from build123d import *

# Parameters (mm, degrees)
BOSS_EXTRUDE1_DEPTH = 5
SKETCH1_3_W         = 10
SKETCH1_3_H         = 5
BOSS_EXTRUDE2_DEPTH = 9
SKETCH2_W           = 40
SKETCH2_H           = 3.955098896
BOSS_EXTRUDE4_DEPTH = 12.5
FILLET1_R           = 2
SKETCH6_R           = 1.6
CUT_EXTRUDE1_DEPTH  = 3.955098897
FILLET2_R           = 1
FILLET3_R           = 2


with BuildPart() as part:
    # Sketch1 → Boss-Extrude1 (new body)
    with BuildSketch(Plane(origin=(0, 0, 0), x_dir=(1, 0, 0), z_dir=(0, 1, 0))):
        Polygon((-4.61462686, -18.720861087), (-14.61462686, -18.720861087), (-14.61462686, -25.920861087), (-34.61462686, -25.920861087), (-34.61462686, -18.720861087), (-44.61462686, -18.720861087), (-44.61462686, -35.875959983), (-4.61462686, -35.875959983), align=None)
    extrude(amount=BOSS_EXTRUDE1_DEPTH)

    # Sketch1<3> → Boss-Extrude2 (add)
    with BuildSketch(Plane(origin=(0, 0, 0), x_dir=(1, 0, 0), z_dir=(0, 1, 0))):
        with Locations((-39.61462686, -21.220861087)):
            Rectangle(SKETCH1_3_W, SKETCH1_3_H)
        with Locations((-9.61462686, -21.220861087)):
            Rectangle(SKETCH1_3_W, SKETCH1_3_H)
    extrude(amount=BOSS_EXTRUDE2_DEPTH)

    # Sketch2 → Boss-Extrude4 (add)
    with BuildSketch(Plane(origin=(0, 5, 0), x_dir=(1, 0, 0), z_dir=(0, 1, 0))):
        with Locations((-24.61462686, -33.898410535)):
            Rectangle(SKETCH2_W, SKETCH2_H)
    extrude(amount=BOSS_EXTRUDE4_DEPTH)

    # Fillet1
    fillet1_edges = [part.edges().sort_by_distance(p)[0] for p in [
        (-34.61462686, 0, 22.320861087),
        (-24.61462686, 0, 25.920861087),
        (-14.61462686, 0, 22.320861087),
        (-9.61462686, 0, 18.720861087),
        (-4.61462686, 0, 27.298410535),
        (-24.61462686, 0, 35.875959983),
        (-44.61462686, 0, 27.298410535),
        (-44.61462686, 4.5, 18.720861087),
        (-34.61462686, 4.5, 18.720861087),
        (-14.61462686, 4.5, 18.720861087),
        (-4.61462686, 4.5, 18.720861087),
        (-4.61462686, 8.75, 35.875959983),
        (-44.61462686, 8.75, 35.875959983),
        (-24.61462686, 5, 25.920861087),
        (-39.61462686, 9, 18.720861087),
        (-44.61462686, 9, 21.220861087),
        (-34.61462686, 9, 21.220861087),
        (-14.61462686, 9, 21.220861087),
        (-4.61462686, 9, 21.220861087),
        (-9.61462686, 9, 18.720861087),
        (-39.61462686, 0, 18.720861087),
    ]]
    fillet(fillet1_edges, radius=FILLET1_R)

    # Sketch6 → Cut-Extrude1 (cut)
    with BuildSketch(Plane(origin=(0, 0, 31.920861087), x_dir=(-1, 0, 0), z_dir=(0, 0, -1))):
        with Locations((24.61462686, 12)):
            Circle(SKETCH6_R)
    extrude(amount=-CUT_EXTRUDE1_DEPTH, mode=Mode.SUBTRACT)

    # Fillet2
    fillet2_edges = [part.edges().sort_by_distance(p)[0] for p in [
        (-23.01462686, 12, 31.920861087),
        (-23.01462686, 12, 35.875959984),
    ]]
    fillet(fillet2_edges, radius=FILLET2_R)

    # Fillet3
    fillet3_edges = [part.edges().sort_by_distance(p)[0] for p in [
        (-24.61462686, 17.5, 31.920861087),
    ]]
    fillet(fillet3_edges, radius=FILLET3_R)


solid = part.part
Design review of the part built by this model. Coordinates are the model's own, in mm. A direction names the side the tool comes from. Round coordinates to 2 decimals unless told otherwise and drop trailing zeros. Write each loop counter-clockwise with the first axis right and the second up, starting at its lowest first coordinate (ties: lowest second). Pieces come first, ordered by that corner, then holes.
Item 1: Consider section B-B on y = 6. Give the boundary of the cut face in (x, z), and give its area (3 significant figures).
Item 2: For pin 1 Ø10 at (x, z) = (-10, 28.5) entering from +Y; pin 2 Ø0.5 at (x, y) = (-23, 2.5) entering from -Z; pin 3 Ø8 at (x, y) = (-18, 13.5) entering from -Z, all flat-tipped, find the tip position at first contact; note any pin that passes through.
Item 3: Consider section D-D on y = 15. Give the boundary of the cut face in (x, z).
Item 4: Consider section C-C on x = -29.5. Give the boundary of the cut face in (y, z), and give its area (3 significant figures).
Item 5: Consider section A-A on y = 12. Give the boundary of the cut face in (x, z), and give its area (3 significant figures).
Item 6: For faces 1 (the cylindrical face through (-5.185, 8.399, 22.2)), 2 (the cylindrical face through (-24.75, 4.4, 26.49)), 3 (the flat face through (-24.5, 2.5, 25.921)), list the 3-axis set-ups (+Z, -Z, +X, -X, +Y, -Y) from which the entire face can be reached by the end or side of a thin tool; tool diameter is ignored.
Item 7: Draft analysis for pull direction X (two halves, no side actions). For faces 4 (the cylindrical face through (-35.185, 0.601, 23.571)), 5 (the cylindrical face through (-44.044, 0.601, 27.206)), 6 (the flat face through (-25, 9, 31.921)), 7 (the cylindrical face through (-5.185, 0.601, 27.39)), state which applies: released by +X, released by -X, zero draft, split by the parting line, or undercut.
Item 8: Wall thickness on L1, parallel to Z at x = -36.5, y = 5.25; L2, parallel to Y at x = -28.5, z = 31.25; L3, parallel to Z at x = -29, y = 6.75: over which ranges is each line inside the solid? List them lowest first.
Check values:
1. outline: (-44.61, 20.72) arc R2 ccw to (-42.61, 18.72) - (-36.61, 18.72) arc R2 ccw to (-34.61, 20.72) - (-34.61, 23.72) - (-44.61, 23.72) - close; (-44.61, 31.92) - (-4.61, 31.92) - (-4.61, 33.88) arc R2 ccw to (-6.61, 35.88) - (-42.61, 35.88) arc R2 ccw to (-44.61, 33.88) - close; (-14.61, 20.72) arc R2 ccw to (-12.61, 18.72) - (-6.61, 18.72) arc R2 ccw to (-4.61, 20.72) - (-4.61, 23.72) - (-14.61, 23.72) - close
1. area: 253 mm2
2. pin 1: stops at y = 17.46
2. pin 2: stops at z = 25.92
2. pin 3: stops at z = 31.92
3. outline: (-44.61, 31.92) - (-4.61, 31.92) - (-4.61, 33.88) arc R2 ccw to (-6.61, 35.88) - (-42.61, 35.88) arc R2 ccw to (-44.61, 33.88) - close
4. outline: (0, 27.92) arc R2 ccw to (2, 25.92) - (3, 25.92) arc R2 ccw to (5, 27.92) - (5, 31.92) - (15.5, 31.92) arc R2 ccw to (17.5, 33.92) - (17.5, 35.88) - (2, 35.88) arc R2 ccw to (0, 33.88) - close
4. area: 95.8 mm2
5. outline: (-44.61, 31.92) - (-27.21, 31.92) arc R1 ccw to (-26.21, 32.92) - (-26.21, 34.88) arc R1 ccw to (-27.21, 35.88) - (-42.61, 35.88) arc R2 ccw to (-44.61, 33.88) - close; (-23.01, 32.92) arc R1 ccw to (-22.01, 31.92) - (-4.61, 31.92) - (-4.61, 33.88) arc R2 ccw to (-6.61, 35.88) - (-22.01, 35.88) arc R1 ccw to (-23.01, 34.88) - close
5. area: 143 mm2
6. face 1: -Z, +X, +Y
6. face 2: -Z, +Y
6. face 3: -Z, +Y, -Y
7. face 4: undercut
7. face 5: released by -X
7. face 6: zero draft
7. face 7: released by +X
8. L1: z = 18.72 to 23.72, 31.92 to 35.88
8. L2: y = 0 to 5
8. L3: z = 31.92 to 35.88
